from build123d import *

# Parameters (mm, degrees)
BASE_FLANGE1_DEPTH         = 1
SKETCHED_START             = 31
SKETCHED_BEND1_DEPTH       = 138
SKETCHED_BEND1_2_DEPTH     = 403
SKETCHED_BEND1_3_OUTLINE_W = 403
SKETCHED_BEND1_3_OUTLINE_H = 1
SKETCHED_BEND1_3_DEPTH     = 29.234623369
SKETCHED_START_2           = 170.765376631
SKETCHED_BEND1_4_OUTLINE_W = 403
SKETCHED_BEND1_4_OUTLINE_H = 1
SKETCHED_BEND1_4_DEPTH     = 29.234623369
SKETCHED_BEND1_5_DEPTH     = 138
SKETCHED_BEND1_6_DEPTH     = 403
SKETCHED_BEND1_7_OUTLINE_W = 138
SKETCHED_BEND1_7_OUTLINE_H = 1
SKETCHED_BEND1_7_DEPTH     = 29.234623369
SKETCHED_START_3           = 435.765376631
SKETCHED_BEND1_8_OUTLINE_W = 138
SKETCHED_BEND1_8_OUTLINE_H = 1
SKETCHED_BEND1_8_DEPTH     = 29.234623369


# Read off the part's stored shape, not the designer's step: Sketched Bend1
# Sheet-metal steps are written as plain solids
with BuildPart() as part:
    # Sketch1 → Base-Flange1 (new body)
    with BuildSketch(Plane.XY):
        Polygon((0, 169), (31, 169), (31, 200), (434, 200), (434, 169), (465, 169), (465, 31), (434, 31), (434, 0), (31, 0), (31, 31), (0, 31), align=None)
    extrude(amount=-BASE_FLANGE1_DEPTH)

    # Sketched Bend1 outline → Sketched Bend1 (add)
    with BuildSketch(Plane(origin=(0, 0, 0), x_dir=(1, 0, 0), z_dir=(0, 1, 0)).offset(SKETCHED_START)):
        with BuildLine():
            Line((29.234623369, -0.7366), (29.234623369, -29.765376631))
            Line((29.234623369, -29.765376631), (30.234623369, -29.765376631))
            Line((30.234623369, -29.765376631), (30.234623369, -0.7366))
            ThreePointArc((30.234623369, -0.7366), (30.450368514, -0.215745145), (30.971223369, 0))
            Line((30.971223369, 0), (29.398582279, 0))
            ThreePointArc((29.398582279, 0), (29.276108612, -0.359286442), (29.234623369, -0.7366))
        make_face()
        with BuildLine():
            Line((435.601417721, 0), (434.028776631, 0))
            ThreePointArc((434.028776631, 0), (434.549631486, -0.215745145), (434.765376631, -0.7366))
            Line((434.765376631, -0.7366), (434.765376631, -29.765376631))
            Line((434.765376631, -29.765376631), (435.765376631, -29.765376631))
            Line((435.765376631, -29.765376631), (435.765376631, -0.7366))
            ThreePointArc((435.765376631, -0.7366), (435.723891388, -0.359286442), (435.601417721, 0))
        make_face()
    extrude(amount=SKETCHED_BEND1_DEPTH)

    # Sketched Bend1 2 outline → Sketched Bend1 2 (add)
    with BuildSketch(Plane.YZ.offset(SKETCHED_START)):
        with BuildLine():
            Line((169.028776631, 0), (170.601417721, 0))
            ThreePointArc((170.601417721, 0), (170.723891388, 0.359286442), (170.765376631, 0.7366))
            Line((170.765376631, 0.7366), (170.765376631, 29.765376631))
            Line((170.765376631, 29.765376631), (169.765376631, 29.765376631))
            Line((169.765376631, 29.765376631), (169.765376631, 0.7366))
            ThreePointArc((169.765376631, 0.7366), (169.549631486, 0.215745145), (169.028776631, 0))
        make_face()
        with BuildLine():
            ThreePointArc((29.234623369, 0.7366), (29.276108612, 0.359286442), (29.398582279, 0))
            Line((29.398582279, 0), (30.971223369, 0))
            ThreePointArc((30.971223369, 0), (30.450368514, 0.215745145), (30.234623369, 0.7366))
            Line((30.234623369, 0.7366), (30.234623369, 29.765376631))
            Line((30.234623369, 29.765376631), (29.234623369, 29.765376631))
            Line((29.234623369, 29.765376631), (29.234623369, 0.7366))
        make_face()
    extrude(amount=SKETCHED_BEND1_2_DEPTH)

    # Sketched Bend1 3 outline → Sketched Bend1 3 (cut)
    with BuildSketch(Plane(origin=(0, 0, 0), x_dir=(1, 0, 0), z_dir=(0, 1, 0))):
        with Locations((232.5, 0.5)):
            Rectangle(SKETCHED_BEND1_3_OUTLINE_W, SKETCHED_BEND1_3_OUTLINE_H)
    extrude(amount=SKETCHED_BEND1_3_DEPTH, mode=Mode.SUBTRACT)

    # Sketched Bend1 4 outline → Sketched Bend1 4 (cut)
    with BuildSketch(Plane(origin=(0, 0, 0), x_dir=(1, 0, 0), z_dir=(0, 1, 0)).offset(SKETCHED_START_2)):
        with Locations((232.5, 0.5)):
            Rectangle(SKETCHED_BEND1_4_OUTLINE_W, SKETCHED_BEND1_4_OUTLINE_H)
    extrude(amount=SKETCHED_BEND1_4_DEPTH, mode=Mode.SUBTRACT)

    # Sketched Bend1 5 outline → Sketched Bend1 5 (cut)
    with BuildSketch(Plane(origin=(0, 0, 0), x_dir=(1, 0, 0), z_dir=(0, 1, 0)).offset(SKETCHED_START)):
        with BuildLine():
            Line((0, 0), (29.398582279, 0))
            ThreePointArc((29.398582279, 0), (30.039397205, 0.728828115), (30.971223369, 1))
            Line((30.971223369, 1), (0, 1))
            Line((0, 1), (0, 0))
        make_face()
        with BuildLine():
            Line((465, 1), (434.028776631, 1))
            ThreePointArc((434.028776631, 1), (434.960602795, 0.728828115), (435.601417721, 0))
            Line((435.601417721, 0), (465, 0))
            Line((465, 0), (465, 1))
        make_face()
    extrude(amount=SKETCHED_BEND1_5_DEPTH, mode=Mode.SUBTRACT)

    # Sketched Bend1 6 outline → Sketched Bend1 6 (cut)
    with BuildSketch(Plane.YZ.offset(SKETCHED_START)):
        with BuildLine():
            ThreePointArc((170.601417721, 0), (169.960602795, -0.728828115), (169.028776631, -1))
            Line((169.028776631, -1), (200, -1))
            Line((200, -1), (200, 0))
            Line((200, 0), (170.601417721, 0))
        make_face()
        with BuildLine():
            Line((0, -1), (30.971223369, -1))
            ThreePointArc((30.971223369, -1), (30.039397205, -0.728828115), (29.398582279, 0))
            Line((29.398582279, 0), (0, 0))
            Line((0, 0), (0, -1))
        make_face()
    extrude(amount=SKETCHED_BEND1_6_DEPTH, mode=Mode.SUBTRACT)

    # Sketched Bend1 7 outline → Sketched Bend1 7 (cut)
    with BuildSketch(Plane.YZ):
        with Locations((100, -0.5)):
            Rectangle(SKETCHED_BEND1_7_OUTLINE_W, SKETCHED_BEND1_7_OUTLINE_H)
    extrude(amount=SKETCHED_BEND1_7_DEPTH, mode=Mode.SUBTRACT)

    # Sketched Bend1 8 outline → Sketched Bend1 8 (cut)
    with BuildSketch(Plane.YZ.offset(SKETCHED_START_3)):
        with Locations((100, -0.5)):
            Rectangle(SKETCHED_BEND1_8_OUTLINE_W, SKETCHED_BEND1_8_OUTLINE_H)
    extrude(amount=SKETCHED_BEND1_8_DEPTH, mode=Mode.SUBTRACT)


solid = part.part
For this review, take the finished solid that the model builds, in its own axes (mm). A direction names the side the tool comes from. Give positions to 0.01 mm unless a question says otherwise; leave off trailing zeros. Loops run counter-clockwise (first coordinate to the right, second up) from the corner with the lowest first, then second, coordinate; pieces in that order, holes last. Notation, with made-up numbers: (-16, -8.5) - (22, -8.5) arc R24 cw to (22, 23.5) - close; hole circle Ø10 at (46.5, 59). An arc over 180 degrees is marked (long way). Write each question's results on one line, items separated by ' | '.
(1) For line 1 along Y through (x, z) = (83.5, 7); line 2 along X through (y, z) = (109.5, 17); line 3 along Z through (x, y) = (240, 161), list the stretches that pass through material, from the lowest coordinate up.
Conclusion:
line 1: 29.23 to 30.23, 169.77 to 170.77 | line 2: 29.23 to 30.23, 434.77 to 435.77 | line 3: -1 to 0
(2) Take a section at A-A (z = 6.5). Give the boundary of the cut face in (x, y).
Conclusion:
outline: (29.23, 31) - (30.23, 31) - (30.23, 169) - (29.23, 169) - close; (31, 29.23) - (434, 29.23) - (434, 30.23) - (31, 30.23) - close; (31, 169.77) - (434, 169.77) - (434, 170.77) - (31, 170.77) - close; (434.77, 31) - (435.77, 31) - (435.77, 169) - (434.77, 169) - close
(3) For faces 4 (the flat face through (230, 29.235, 15)), 5 (the flat face through (230, 30.235, 15)), 6 (the flat face through (434.765, 99, 15)), list the 3-axis set-ups (+Z, -Z, +X, -X, +Y, -Y) from which the entire face can be reached by the end or side of a thin tool; tool diameter is ignored.
Conclusion:
face 4: +Z, -Z, +X, -X, -Y | face 5: +Z, +X, -X | face 6: +Z, +Y, -Y
(4) Take a section at C-C (y = 48). Give the boundary of the cut face in (x, z).
Conclusion:
outline: (29.23, 0.74) arc R1.74 ccw to (30.97, -1) - (434.03, -1) arc R1.74 ccw to (435.77, 0.74) - (435.77, 29.77) - (434.77, 29.77) - (434.77, 0.74) arc R0.74 cw to (434.03, 0) - (30.97, 0) arc R0.74 cw to (30.23, 0.74) - (30.23, 29.77) - (29.23, 29.77) - close
(5) For pin 1 Ø6 at (x, y) = (321, 66) entering from +Z; pin 2 Ø0.9 at (y, z) = (30.5, 11.5) entering from -X; pin 3 Ø1.4 at (x, z) = (30, 14) entering from +Y, all flat-tipped, find the tip position at first contact; note any pin that passes through.
Conclusion:
pin 1: z = 0 | pin 2: x = 31 | pin 3: y = 169
(6) Draft analysis for pull direction X (two halves, no side actions). For faces 1 (the flat face through (235, 101, 0)), 2 (the flat face through (235, 101, -1)), 3 (the flat face through (435.765, 99, 15)), state which applies: +X half, -X half, draft (parallel to the pull), parting line (faces both ways), or undercut.
Conclusion:
face 1: undercut | face 2: draft | face 3: +X half
(7) Take a section at B-B (x = 215). Give the boundary of the cut face in (y, z), then the cut area to 3 significant figures.
Conclusion:
outline: (29.23, 0.74) arc R1.74 ccw to (30.97, -1) - (169.03, -1) arc R1.74 ccw to (170.77, 0.74) - (170.77, 29.77) - (169.77, 29.77) - (169.77, 0.74) arc R0.74 cw to (169.03, 0) - (30.97, 0) arc R0.74 cw to (30.23, 0.74) - (30.23, 29.77) - (29.23, 29.77) - close | area: 200 mm^2
